Drawing for the job (mm, zero at the part's lowest x, y, z). Give positions to 0.01 mm unless a question says otherwise; leave off trailing zeros. Loops run counter-clockwise (first coordinate to the right, second up) from the corner with the lowest first, then second, coordinate; pieces in that order, holes last.
1) Band-saw the part on A-A on x = 55. List the corners of the cut face in (y, z).
2) Wall check: line 1 (Y direction, x = 55, z = 1.35); line 2 (Y direction, x = 57.5, z = 1.5) (1 decimal); line 3 (X direction, y = 28, z = 0.3) (1 decimal). Give the ranges that are in metal, low to high.
3) Band-saw the part on D-D on y = 24.5. List the corners of the cut face in (x, z) (1 decimal).
4) Band-saw the part on C-C on x = 43. List the corners of the cut face in (y, z) (1 decimal).
5) Flat gauge pins, fed straight in: P1, Ø1.5, axis at x = 26.5, y = 58, coming from the -Z side; P2, Ø6.5, axis at x = 55, y = 15, coming from the +Z side. Where does each tip first touch, or does it go through?
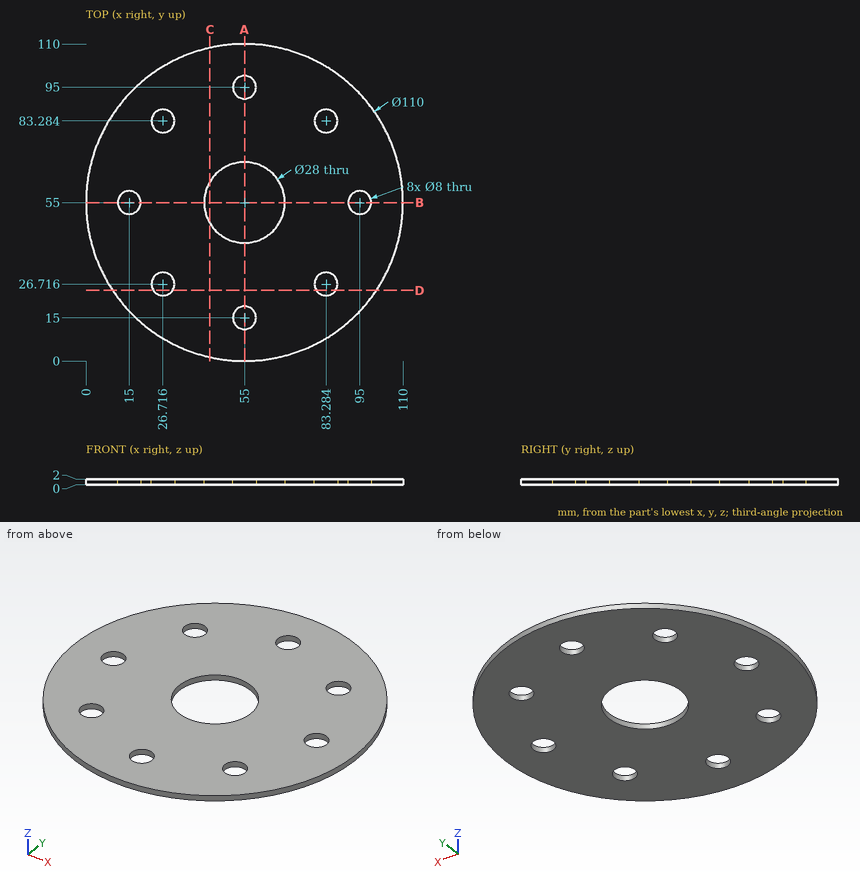
Findings below:
1. outline: (0, 0) - (11, 0) - (11, 2) - (0, 2) - close; (19, 0) - (41, 0) - (41, 2) - (19, 2) - close; (69, 0) - (91, 0) - (91, 2) - (69, 2) - close; (99, 0) - (110, 0) - (110, 2) - (99, 2) - close
2. line 1: y = 0 to 11, 19 to 41, 69 to 91, 99 to 110
2. line 2: y = 0.1 to 11.9, 18.1 to 41.2, 68.8 to 91.9, 98.1 to 109.9
2. line 3: x = 7.1 to 22.9, 30.5 to 79.5, 87.1 to 102.9
3. outline: (9.2, 0) - (23.4, 0) - (23.4, 2) - (9.2, 2) - close; (30, 0) - (80, 0) - (80, 2) - (30, 2) - close; (86.6, 0) - (100.8, 0) - (100.8, 2) - (86.6, 2) - close
4. outline: (1.3, 0) - (47.8, 0) - (47.8, 2) - (1.3, 2) - close; (62.2, 0) - (108.7, 0) - (108.7, 2) - (62.2, 2) - close
5. P1: stops at z = 0
5. P2: passes through
